For this review, take the finished solid that the model builds, in its own axes (mm). A direction names the side the tool comes from. Coordinates: 2 decimals unless noted, no trailing zeros. Loops run counter-clockwise (first coordinate to the right, second up) from the corner with the lowest first, then second, coordinate; pieces in that order, holes last. Notation, with made-up numbers: (89, 39.25) - (138, 39.25) arc R13 ccw to (138, 56.25) - close; hole circle Ø8 at (87, 17.25). An arc over 180 degrees is marked (long way). One line per item, written item: value. Start each with the question number.
1. Take a section at C-C, the plane x = -9. State the section outline as (y, z) points, and give its area (3 significant figures).
2. To check wall thickness, follow line 1 (Z direction, x = 0.55, y = -10); line 2 (X direction, y = -11.5, z = 165.5); line 3 (Y direction, x = 0.4, z = 100). State the ranges of each line that lie inside material, in increasing order. Write a range as from..to.
3. Insertion check: pin 1 (1.9 mm diameter, centred on y = -10, z = 185, fed in from -X) (1 decimal); pin 2 (8 mm diameter, centred on x = -10.5, z = 82.5, fed in from -Y); pin 3 (1.5 mm diameter, centred on y = -3.5, z = 124, fed in from -X). Each pin has a flat end and moves straight along its axis. Give the tip position at first contact, or say it passes through.
4. Take a section at B-B, the plane y = -6. State the section outline as (x, z) points.
5. The part is to be moulded in two halves that separate along Y. For faces 1 (the face through (0, 0, 0)), 2 (the face through (0.74, -10.07, 101.6)), 3 (the face through (-7, 7, 99)), say which applies: released by +Y, released by -Y, zero draft, split by the parting line, or undercut.
6. Take a section at A-A, the plane z = 77. State the section outline as (x, y) points, and give its area (3 significant figures).
7. For faces 4 (the face through (0, -8, 99)), 5 (the face through (0.74, -10.07, 16.6)), list the 3-axis set-ups (+Z, -Z, +X, -X, +Y, -Y) from which the entire face can be reached by the end or side of a thin tool; tool diameter is ignored.
Autodesk Inventor part; units mm, degrees
ref_plane "YZ Plane" through (0, 0, 0) normal (1, 0, 0) x (0, 1, 0)
ref_plane "XZ Plane" through (0, 0, 0) normal (0, 1, 0) x (-1, 0, 0)
ref_plane "XY Plane" through (0, 0, 0) normal (0, 0, 1) x (1, 0, 0)
sketch "Skizze1" plane through (0, 0, 0) normal (0, 0, 1) x (1, 0, 0)
  line L0 (0, -0.8284) -> (0, -20)
  line L1 (0, 0) -> (19.1716, 0) construction
  line L2 (0, -20) -> (1.5, -20)
  line L3 (1.5, -20) -> (1.5, 1.5)
  line L4 (-0.5858, 0.5858) -> (-14.1421, 14.1421)
  line L5 (-14.1421, 14.1421) -> (-13.0815, 15.2028)
  line L6 (-13.0815, 15.2028) -> (1.5, 1.5)
  arc A0 (0, -0.8284) -> (-0.5858, 0.5858) centre (-2, -0.8284) ccw
  dimension "d0" = 20
  dimension "d1" = 90
  dimension "d2" = 1.5
  dimension "d3" = 90
  dimension "d4" = 21.5
  dimension "d5" = 20
  dimension "d6" = 135
  dimension "d7" = 2
extrude "Extrusion1" add sketch "Skizze1" along normal blind 200
hole "Bohrung1" at (1.5, -10, 185) direction (-1, 0, 0) diameter 3.2 end through all
pattern_linear "Rechteckige Anordnung1" count 3 spacing 85 along (0, 0, -1) of "Bohrung1"
fillet "Rundung1" radius 0.69 5 edges at (1.5, -20, 100) (0, -20, 100) (-14.1421, 14.1421, 100) (1.5, 1.5, 100) (-13.0815, 15.2028, 100)
properties part number "LED strip mount" material "ABS-Kunststoff"
Solutions:
1. outline: (9, 0) - (11.37, 0) - (11.37, 200) - (9, 200) - close
1. area: 473 mm2
2. line 1: 0..13.4, 16.6..98.4, 101.6..183.4, 186.6..200
2. line 2: 0..1.5
2. line 3: -19.94..-11.6, -8.4..2.53
3. pin 1: through
3. pin 2: y = 6.5
3. pin 3: x = 0
4. outline: (0, 0) - (1.5, 0) - (1.5, 200) - (0, 200) - close
5. face 1: zero draft
5. face 2: undercut
5. face 3: released by -Y
6. outline: (-13.65, 13.65) - (-0.59, 0.59) arc R2 cw to (0, -0.83) - (0, -19.31) arc R0.69 ccw to (0.69, -20) - (0.81, -20) arc R0.69 ccw to (1.5, -19.31) - (1.5, 1.2) arc R0.69 ccw to (1.28, 1.7) - (-12.59, 14.74) arc R0.69 ccw to (-13.55, 14.73) - (-13.65, 14.63) arc R0.69 ccw to start
6. area: 67.0 mm2
7. face 4: +Z, -Z, -X, -Y
7. face 5: +X, -X
